from build123d import *

# Parameters (mm, degrees)
SKETCH1_R           = 4
BOSS_EXTRUDE1_DEPTH = 2.3
SKETCH2_R           = 2
BOSS_EXTRUDE2_DEPTH = 5.7
CHAMFER1_SIZE       = 0.3
CUT_EXTRUDE1_DEPTH  = 2
CHAMFER2_SIZE       = 2.4


with BuildPart() as part:
    # Sketch1 → Boss-Extrude1 (new body)
    with BuildSketch(Plane.XY):
        Circle(SKETCH1_R)
    extrude(amount=BOSS_EXTRUDE1_DEPTH)

    # Sketch2 → Boss-Extrude2 (add)
    with BuildSketch(Plane(origin=(0, 0, 0), x_dir=(-1, 0, 0), z_dir=(0, 0, -1))):
        with Locations(Location((0, 0, 0), (0, 0, 180))):
            Circle(SKETCH2_R)
    extrude(amount=BOSS_EXTRUDE2_DEPTH)

    # Chamfer1
    chamfer1_edges = [part.edges().sort_by_distance(p)[0] for p in [
        (-2, 0, -5.7),
    ]]
    chamfer(chamfer1_edges, length=CHAMFER1_SIZE)

    # Sketch3 → Cut-Extrude1 (cut)
    with BuildSketch(Plane.XY.offset(2.3)):
        Polygon((0, 1.443375673), (-1.25, 0.721687836), (-1.25, -0.721687836), (0, -1.443375673), (1.25, -0.721687836), (1.25, 0.721687836), align=None)
    extrude(amount=-CUT_EXTRUDE1_DEPTH, mode=Mode.SUBTRACT)

    # Chamfer2
    # the kernel refuses this chamfer: 2.4 mm, written as the material it takes off along each edge
    with BuildSketch(Plane(origin=(0, 0, 0), x_dir=(1, 0, 0), z_dir=(0, -1, 0))) as chamfer2_piece_1_section:
        Polygon((4 - CHAMFER2_SIZE, 0), (4, CHAMFER2_SIZE), (4, 0), align=None)
    chamfer2_piece_1 = revolve(axis=Axis((0, 0, 0), (0, 0, 1)), mode=Mode.PRIVATE)
    chamfer2_piece_1 = chamfer2_piece_1 - Plane(origin=(0, 0, 1.405884102), x_dir=(1, 0, 0), z_dir=(0, 0, 1)) * Cylinder(2, 16, mode=Mode.PRIVATE)
    add(chamfer2_piece_1, mode=Mode.SUBTRACT)


solid = part.part
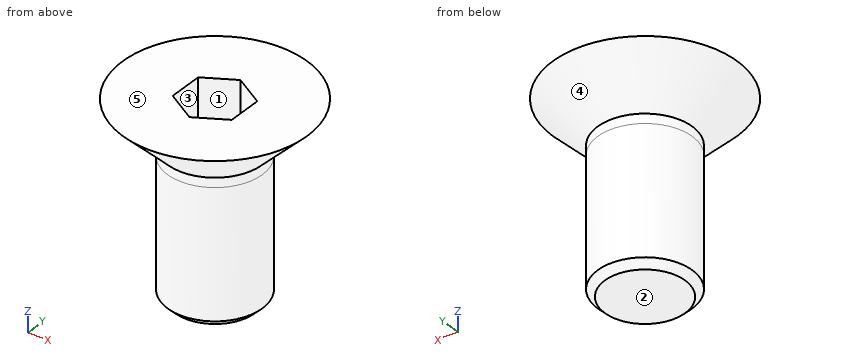
Geometry check sheet. Reference: the model listing, model coordinates, mm. Face numbers are marked on the shaded views. A direction names the side the tool comes from. Give positions to 0.01 mm unless a question says otherwise; leave off trailing zeros. Write each loop counter-clockwise with the first axis right and the second up, starting at its lowest first coordinate (ties: lowest second). Pieces come first, ordered by that corner, then holes. Notation, with made-up numbers: (8, 15) - (40, 15) arc R15 cw to (40, 44) - close; hole circle Ø9 at (7, 67.5). An arc over 180 degrees is marked (long way). Put each result on its own line as item: value.
1. Draft check along X on the marked faces 3, 4 and 5. Enter one of: +X half, -X half, draft (parallel to the pull), parting line (faces both ways), or undercut.
Ans:
face 3: undercut
face 4: parting line
face 5: draft
2. Go/stop test with flat-tipped pins: pin 1 (2 mm diameter, centred on x = 0, y = 0, fed in from +Z); pin 2 (1.2 mm diameter, centred on y = 0.5, z = 1.5, fed in from -X); pin 3 (1.5 mm diameter, centred on x = 0, z = -4.5, fed in from -Y). Record where each tip stops, or that it passes through.
Ans:
pin 1: stops at z = 0.3
pin 2: stops at x = -3.67
pin 3: stops at y = -2
3. Sectioned sample at A-A, the plane z = 1.5. Enter the section's corners in (x, y).
Ans:
outline: circle Ø6.2 at (0, 0); hole (-1.25, -0.72) - (0, -1.44) - (1.25, -0.72) - (1.25, 0.72) - (0, 1.44) - (-1.25, 0.72) - close
4. Thickness scan on line 1 (Z direction, x = 1.75, y = -1.75); line 2 (Y direction, x = -1.25, z = -0.5); line 3 (Z direction, x = -2.75, y = -0.25). Record the ranges inside material, lowest first.
Ans:
line 1: z = 0.87 to 2.3
line 2: y = -1.56 to 1.56
line 3: z = 1.16 to 2.3
5. Set-up check for the marked faces 1 and 2: record each of +Z, -Z, +X, -X, +Y, -Y from which the full face is reachable in a straight line by a thin tool's end or side.
Ans:
face 1: +Z
face 2: -Z, +X, -X, +Y, -Y
6. Sectioned sample at B-B, the plane y = 0. Enter the section's corners in (x, z), plus the area to 3 significant figures.
Ans:
outline: (-3.9, 2.3) - (-2, 0.4) - (-2, -5.4) - (-1.7, -5.7) - (1.7, -5.7) - (2, -5.4) - (2, 0.4) - (3.9, 2.3) - (1.25, 2.3) - (1.25, 0.3) - (-1.25, 0.3) - (-1.25, 2.3) - close
area: 30.5 mm²
7. Sectioned sample at C-C, the plane z = -4.25. Enter the section's corners in (x, y), plus the area to 3 significant figures.
Ans:
outline: circle Ø4 at (0, 0)
area: 12.6 mm²
